from build123d import *

# Parameters (mm, degrees)
SCHIZZO1_W                   = 70
SCHIZZO1_H                   = 167
ESTRUSIONE_ESTRUSIONE1_DEPTH = 20
SCHIZZO2_R                   = 3
TAGLIO_ESTRUSIONE1_DEPTH     = 20


with BuildPart() as part:
    # Schizzo1 → Estrusione-Estrusione1 (new body)
    with BuildSketch(Plane.XY):
        Rectangle(SCHIZZO1_W, SCHIZZO1_H)
    extrude(amount=ESTRUSIONE_ESTRUSIONE1_DEPTH)

    # Schizzo2 → Taglio-Estrusione1 (cut)
    with BuildSketch(Plane(origin=(0, 0, 0), x_dir=(-1, 0, 0), z_dir=(0, 0, -1))):
        with Locations((-28.5, 65.5)):
            Circle(SCHIZZO2_R)
        with Locations((28.5, 65.5)):
            Circle(SCHIZZO2_R)
        with Locations((-28.5, 20.5)):
            Circle(SCHIZZO2_R)
        with Locations((28.5, 20.5)):
            Circle(SCHIZZO2_R)
        with Locations((-28.5, -20.5)):
            Circle(SCHIZZO2_R)
        with Locations((28.5, -20.5)):
            Circle(SCHIZZO2_R)
        with Locations((-28.5, -65.5)):
            Circle(SCHIZZO2_R)
        with Locations((28.5, -65.5)):
            Circle(SCHIZZO2_R)
    extrude(amount=-TAGLIO_ESTRUSIONE1_DEPTH, mode=Mode.SUBTRACT)


solid = part.part
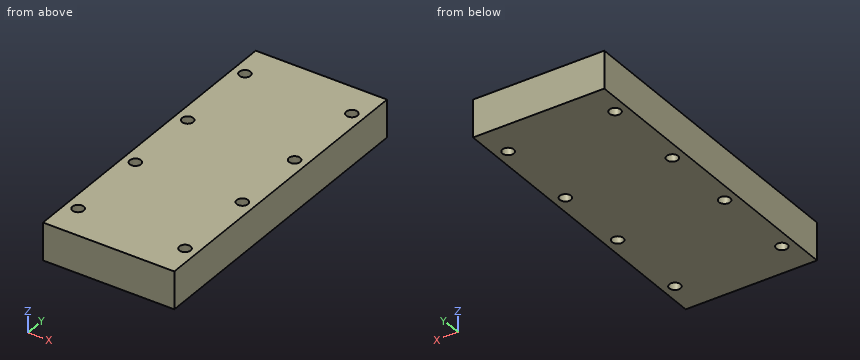
Read the model definition and answer for the solid it produces. Units are mm, in the model's axes. Round coordinates to 2 decimals unless told otherwise and drop trailing zeros. Write each loop counter-clockwise with the first axis right and the second up, starting at its lowest first coordinate (ties: lowest second). Pieces come first, ordered by that corner, then holes.
Q1. Straight lines are drawn through the part: line 1 (Y direction, x = 28.5, z = 7.25); line 2 (X direction, y = -20, z = 11.25); line 3 (Y direction, x = -30, z = 1.75). For each, find the intervals that lie inside material, in ascending order.
Values:
line 1: y = -83.5 to -68.5, -62.5 to -23.5, -17.5 to 17.5, 23.5 to 62.5, 68.5 to 83.5
line 2: x = -35 to -31.46, -25.54 to 25.54, 31.46 to 35
line 3: y = -83.5 to -68.1, -62.9 to -23.1, -17.9 to 17.9, 23.1 to 62.9, 68.1 to 83.5
Q2. Find section B-B on z = 9. State how many separate pieces and enclosed holes the cut face has, and give its area (3 significant figures).
Values:
separate pieces: 1
enclosed holes: 8
area: 11,500 mm2
Q3. Find section A-A on x = 28.5. Determine the outline of the cut face in (y, z).
Values:
outline: (-83.5, 0) - (-68.5, 0) - (-68.5, 20) - (-83.5, 20) - close; (-62.5, 0) - (-23.5, 0) - (-23.5, 20) - (-62.5, 20) - close; (-17.5, 0) - (17.5, 0) - (17.5, 20) - (-17.5, 20) - close; (23.5, 0) - (62.5, 0) - (62.5, 20) - (23.5, 20) - close; (68.5, 0) - (83.5, 0) - (83.5, 20) - (68.5, 20) - close
Q4. Find section D-D on y = 67. Determine the outline of the cut face in (x, z), and give its area (3 significant figures).
Values:
outline: (-35, 0) - (-31.1, 0) - (-31.1, 20) - (-35, 20) - close; (-25.9, 0) - (25.9, 0) - (25.9, 20) - (-25.9, 20) - close; (31.1, 0) - (35, 0) - (35, 20) - (31.1, 20) - close
area: 1,190 mm2
Q5. Find section C-C on y = -65.5. Determine the outline of the cut face in (x, z), and give its area (3 significant figures).
Values:
outline: (-35, 0) - (-31.5, 0) - (-31.5, 20) - (-35, 20) - close; (-25.5, 0) - (25.5, 0) - (25.5, 20) - (-25.5, 20) - close; (31.5, 0) - (35, 0) - (35, 20) - (31.5, 20) - close
area: 1,160 mm2
